Verification items for the finished model (mm, model axes). Face numbers are marked on the shaded views. A direction names the side the tool comes from. Round coordinates to 2 decimals unless told otherwise and drop trailing zeros. Order: outer loops, then holes, each group sorted by start corner. A loop starts at its lowest first (then second) coordinate and runs counter-clockwise, first axis right, second up. Notation, with made-up numbers: (56.25, -15) -> (76.25, -15) arc R13 cw to (76.25, 0) -> close; hole circle Ø9 at (81.25, -13.5). An arc over 180 degrees is marked (long way). Write item = value, one per line. Start each with the question number.
from build123d import *

# Parameters (mm, degrees)
SKETCH1_W           = 125
SKETCH1_H           = 52
BOSS_EXTRUDE1_DEPTH = 30
SKETCH2_W           = 24.62687601
SKETCH2_H           = 18.598470566
BOSS_EXTRUDE2_DEPTH = 31
SKETCH3_R           = 6.039414619
BOSS_EXTRUDE3_DEPTH = 19.05
BOSS_EXTRUDE4_DEPTH = 2.54


with BuildPart() as part:
    # Sketch1 → Boss-Extrude1 (new body)
    with BuildSketch(Plane(origin=(0, 0, 0), x_dir=(1, 0, 0), z_dir=(0, 1, 0))):
        Rectangle(SKETCH1_W, SKETCH1_H)
    extrude(amount=BOSS_EXTRUDE1_DEPTH)

    # Sketch2 → Boss-Extrude2 (add)
    with BuildSketch(Plane(origin=(62.5, 0, 0), x_dir=(0, 0, -1), z_dir=(1, 0, 0))):
        with Locations((0, 15)):
            Rectangle(SKETCH2_W, SKETCH2_H)
    extrude(amount=BOSS_EXTRUDE2_DEPTH)

    # Sketch3 → Boss-Extrude3 (add)
    with BuildSketch(Plane.ZY.offset(62.5)):
        with Locations(Location((0, 15, 0), (0, 0, 180))):
            Circle(SKETCH3_R)
    extrude(amount=BOSS_EXTRUDE3_DEPTH)

    # Sketch4 → Boss-Extrude4 (add)
    # profile 1 of 3: a face of its own
    with BuildSketch(Plane(origin=(0, 30, 0), x_dir=(1, 0, 0), z_dir=(0, 1, 0))):
        with BuildLine():
            Line((-20.314153968, 0.487864775), (-21.453897558, 0.487864775))
            add(Edge.make_bspline(
                [(-21.453897558, 0.487864775), (-21.446469317, 0.639070568), (-21.431880449, 0.936034721), (-21.363560657, 1.369010039), (-21.26580376, 1.782866023), (-21.127586198, 2.17427971), (-20.95593199, 2.546711954), (-20.750083034, 2.898683439), (-20.506265347, 3.228851467), (-20.22974377, 3.53415527), (-19.929411851, 3.814235884), (-19.60535887, 4.056099193), (-19.264835486, 4.260451887), (-18.908874809, 4.431289536), (-18.533460764, 4.559522691), (-18.142000109, 4.654669783), (-17.732772957, 4.71191538), (-17.453953448, 4.71806866), (-17.312150763, 4.721198109)],
                knots=[0, 0, 0, 0, 1.10065271, 2.161652631, 3.183658789, 4.190468796, 5.17591951, 6.163126047, 7.15150782, 8.156236427, 9.156009102, 10.134482811, 11.092018607, 12.041330605, 13.001268258, 13.972401359, 14.968799086, 16, 16, 16, 16], degree=3))
            add(Edge.make_bspline(
                [(-17.312150763, 4.721198109), (-17.17289318, 4.717937995), (-16.899257003, 4.711531989), (-16.499889122, 4.656519111), (-16.119697225, 4.570356536), (-15.759424473, 4.449469168), (-15.421945324, 4.286965675), (-15.104724562, 4.091757463), (-14.80398562, 3.865988361), (-14.533269577, 3.600181666), (-14.284683118, 3.316418728), (-14.070226364, 3.013476906), (-13.886572885, 2.700587784), (-13.733491875, 2.375365452), (-13.620802456, 2.034747721), (-13.535247244, 1.683693585), (-13.486887772, 1.318569271), (-13.479465807, 1.071439769), (-13.47569243, 0.945797468)],
                knots=[0, 0, 0, 0, 1.111607364, 2.184268762, 3.212621178, 4.221274766, 5.211760367, 6.196651075, 7.1921475, 8.207485113, 9.220403448, 10.201281604, 11.166441695, 12.114753415, 13.065576456, 14.026450734, 14.996634279, 16, 16, 16, 16], degree=3))
            add(Edge.make_bspline(
                [(-13.47569243, 0.945797468), (-13.481836555, 0.768912468), (-13.494016985, 0.41824655), (-13.598209151, -0.097064524), (-13.76093792, -0.596332073), (-13.956871186, -0.998150283), (-14.15452834, -1.321940389), (-14.332645868, -1.588526833), (-14.541161039, -1.875566675), (-14.783108732, -2.182098728), (-15.053484011, -2.510524012), (-15.354735861, -2.860644127), (-15.689012495, -3.228841692), (-15.923630484, -3.480322017), (-16.045203648, -3.610632821)],
                knots=[0, 0, 0, 0, 1.184426356, 2.348067706, 3.509069118, 4.696110526, 5.333549288, 6.050745305, 6.844228056, 7.710549037, 8.667450064, 9.695053472, 10.805634456, 12, 12, 12, 12], degree=3))
            Line((-16.045203648, -3.610632821), (-19.222747718, -7.001878814))
            Line((-19.222747718, -7.001878814), (-13.312871917, -7.001878814))
            Line((-13.312871917, -7.001878814), (-13.312871917, -8.304442917))
            Line((-13.312871917, -8.304442917), (-21.942359096, -8.304442917))
            Line((-21.942359096, -8.304442917), (-17.017038583, -3.048393237))
            add(Edge.make_bspline(
                [(-17.017038583, -3.048393237), (-16.897121966, -2.923213668), (-16.666786684, -2.682769334), (-16.341004191, -2.331730593), (-16.048399862, -2.006067973), (-15.787079609, -1.706396783), (-15.562712318, -1.428333666), (-15.363604505, -1.180884313), (-15.204072217, -0.953175307), (-15.030933496, -0.689230794), (-14.863242763, -0.366968957), (-14.719143643, 0.026853286), (-14.631278336, 0.432263603), (-14.620737932, 0.706228138), (-14.615436019, 0.844034647)],
                knots=[0, 0, 0, 0, 1.329631726, 2.553950428, 3.673215718, 4.687767853, 5.603093632, 6.413772471, 7.123043292, 7.734684054, 8.834405432, 9.900288307, 10.943827018, 12, 12, 12, 12], degree=3))
            add(Edge.make_bspline(
                [(-14.615436019, 0.844034647), (-14.617742856, 0.930690007), (-14.622289187, 1.101471081), (-14.662412832, 1.351863407), (-14.723048097, 1.593398589), (-14.809935176, 1.826819578), (-14.92462249, 2.049779515), (-15.064225898, 2.262549801), (-15.225298413, 2.46824976), (-15.411630162, 2.661120299), (-15.616323391, 2.83776353), (-15.832565383, 2.994242354), (-16.061347189, 3.125012842), (-16.301704204, 3.232213532), (-16.552966336, 3.316307058), (-16.815619554, 3.37457676), (-17.088938127, 3.411161774), (-17.27556824, 3.416111769), (-17.370664385, 3.418634006)],
                knots=[0, 0, 0, 0, 0.991446411, 1.95395049, 2.89581595, 3.838931463, 4.798493298, 5.75982156, 6.748411868, 7.785213223, 8.824556874, 9.840280684, 10.836137867, 11.835679398, 12.848801643, 13.863922112, 14.911575587, 16, 16, 16, 16], degree=3))
            add(Edge.make_bspline(
                [(-17.370664385, 3.418634006), (-17.469981406, 3.416039461), (-17.665023638, 3.410944201), (-17.951386986, 3.375301963), (-18.224566808, 3.313812771), (-18.485250284, 3.229714553), (-18.733878496, 3.122822104), (-18.969242313, 2.989683488), (-19.190813368, 2.830811955), (-19.399008181, 2.650687651), (-19.590828905, 2.450145212), (-19.759364712, 2.226589061), (-19.906626706, 1.984101011), (-20.035111639, 1.723335356), (-20.139453714, 1.441925925), (-20.21918486, 1.140871682), (-20.282274275, 0.821479812), (-20.303350907, 0.60091679), (-20.314153968, 0.487864775)],
                knots=[0, 0, 0, 0, 1.031018746, 2.02475058, 2.990194455, 3.934040569, 4.864654155, 5.795059489, 6.735614925, 7.690564532, 8.649604399, 9.611025574, 10.590972636, 11.591080095, 12.624614302, 13.701020113, 14.821632451, 16, 16, 16, 16], degree=3))
        make_face()
    # profile 2 of 3: a face of its own
    with BuildSketch(Plane(origin=(0, 30, 0), x_dir=(1, 0, 0), z_dir=(0, 1, 0))):
        Polygon((-5.24053618, 4.721198109), (-5.009025763, 4.721198109), (-5.009025763, -4.071109584), (-3.543641148, -4.071109584), (-3.543641148, -5.373673686), (-5.009025763, -5.373673686), (-5.009025763, -8.304442917), (-6.148769353, -8.304442917), (-6.148769353, -5.373673686), (-12.173128327, -5.373673686), align=None)
        Polygon((-6.148769353, -4.071109584), (-6.148769353, 1.444435288), (-9.934346276, -4.071109584), align=None, mode=Mode.SUBTRACT)
    # profile 3 of 3: a face of its own
    with BuildSketch(Plane(origin=(0, 30, 0), x_dir=(1, 0, 0), z_dir=(0, 1, 0))):
        Polygon((2.64353834, 4.395557083), (3.864692186, 4.395557083), (8.098025519, -5.612816314), (12.331358852, 4.395557083), (13.552512699, 4.395557083), (8.179435776, -8.304442917), (8.016615263, -8.304442917), align=None)
    extrude(amount=BOSS_EXTRUDE4_DEPTH)


solid = part.part
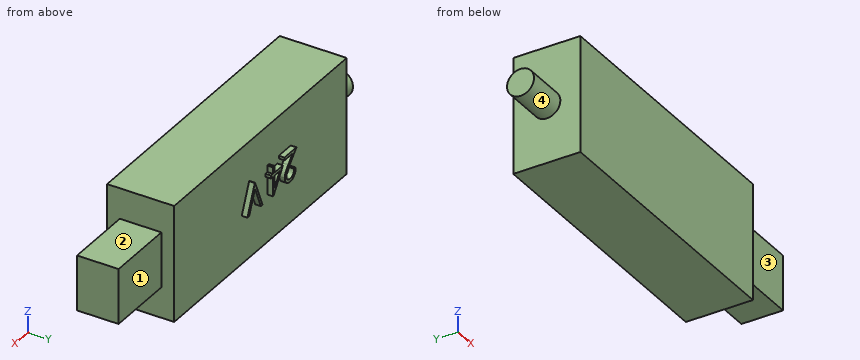
(1) Scan lines: line 1 along Z through (x, y) = (69.5, 23.5); line 2 along X through (y, z) = (8, 20); line 3 along X through (y, z) = (6, -8). Record each from-to range of solid material in increasing order. Write a range as from..to.
(2) Depth check by flat-ended pin: pin 1 (1 mm diameter, centred on y = 29, z = 7.5, fed in from +X); pin 2 (12.5 mm diameter, centred on x = 82, z = 5, fed in from +Y); pin 3 (7.5 mm diameter, centred on x = 72, z = -3.5, fed in from -Y). Enter the tip coordinate at first touch or a pass-through.
(3) Set-up check for the marked faces 1, 2, 3 and 4: record each of +Z, -Z, +X, -X, +Y, -Y from which the full face is reachable in a straight line by a thin tool's end or side.
(4) Cross-section at C-C (z = 16). Enter the section's corners in (x, y).
(5) Cross-section at B-B (x = 51). Enter the section's corners in (y, z), and give its area (3 significant figures).
(6) Cross-section at A-A (y = 15). Enter the section's corners in (x, z).
Outcome:
q1.line_1 = -12.31..12.31
q1.line_2 = -62.5..62.5
q1.line_3 = -62.5..93.5
q2.pin_1 = 62.5
q2.pin_2 = 24.3
q2.pin_3 = 5.7
q3.face_1 = +Z, -Z, +X, +Y
q3.face_2 = +Z, +X, +Y, -Y
q3.face_3 = +Z, -Z, +X, -Y
q3.face_4 = -X
q4.outline = (-62.5, 0) -> (62.5, 0) -> (62.5, 30) -> (-62.5, 30) -> close
q5.outline = (0, -26) -> (30, -26) -> (30, 26) -> (0, 26) -> close
q5.area = 1,560 mm^2
q6.outline = (-81.55, -6.04) -> (-62.5, -6.04) -> (-62.5, -26) -> (62.5, -26) -> (62.5, -12.31) -> (93.5, -12.31) -> (93.5, 12.31) -> (62.5, 12.31) -> (62.5, 26) -> (-62.5, 26) -> (-62.5, 6.04) -> (-81.55, 6.04) -> close
